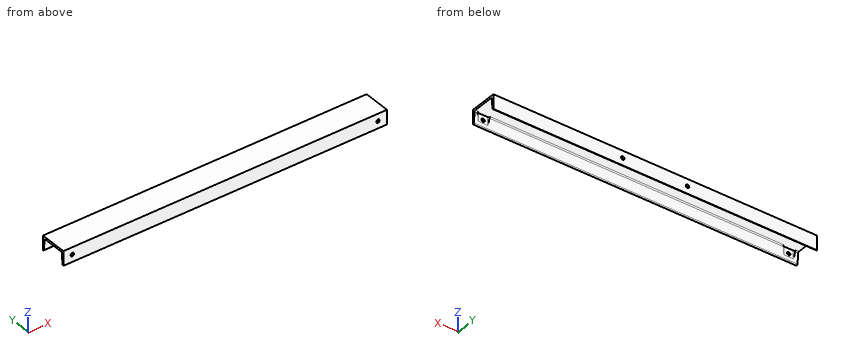
```python
from build123d import *

# Parameters (mm, degrees)
STRUCTURAL_MEMBER1_DEPTH = 900
SKETCH12_R               = 4.7625
CUT_EXTRUDE1_DEPTH       = 454.327971782
CUT_EXTRUDE2_DEPTH       = 40
SKETCH18_R               = 4.7625
CUT_EXTRUDE3_DEPTH       = 10


with BuildPart() as part:
    # Sketch17 → Structural Member1 (new body)
    with BuildSketch(Plane(origin=(-450, 0, 0), x_dir=(0, 0, 1), z_dir=(1, 0, 0))):
        with BuildLine():
            Line((0, 37.5), (0, -37.5))
            Line((0, -37.5), (-40, -37.5))
            Line((-40, -37.5), (-40, -37.246949676))
            ThreePointArc((-40, -37.246949676), (-39.212582687, -35.220998578), (-37.263681431, -34.258560126))
            Line((-37.263681431, -34.258560126), (-8.736318569, -31.741439874))
            ThreePointArc((-8.736318569, -31.741439874), (-6.787417313, -30.779001422), (-6, -28.753050324))
            Line((-6, -28.753050324), (-6, 28.753050324))
            ThreePointArc((-6, 28.753050324), (-6.787417313, 30.779001422), (-8.736318569, 31.741439874))
            Line((-8.736318569, 31.741439874), (-37.263681431, 34.258560126))
            ThreePointArc((-37.263681431, 34.258560126), (-39.212582687, 35.220998578), (-40, 37.246949676))
            Line((-40, 37.246949676), (-40, 37.5))
            Line((-40, 37.5), (0, 37.5))
        make_face()
    extrude(amount=STRUCTURAL_MEMBER1_DEPTH)

    # Sketch12 → Cut-Extrude1 (cut, through all)
    with BuildSketch(Plane(origin=(0, 0, 0), x_dir=(1, 0, 0), z_dir=(0, 1, 0))):
        with Locations(Location((-425, 20, 0), (0, 0, 270))):
            Circle(SKETCH12_R)
        with Locations(Location((425, 20, 0), (0, 0, 270))):
            Circle(SKETCH12_R)
    extrude(amount=-CUT_EXTRUDE1_DEPTH, mode=Mode.SUBTRACT)

    # Sketch15 → Cut-Extrude2 (cut)
    with BuildSketch(Plane(origin=(0, 0, -6), x_dir=(-1, 0, 0), z_dir=(0, 0, -1))):
        with BuildLine():
            Line((-412.5, -33.5), (-437.5, -33.5))
            ThreePointArc((-437.5, -33.5), (-442.5, -28.5), (-437.5, -23.5))
            Line((-437.5, -23.5), (-412.5, -23.5))
            ThreePointArc((-412.5, -23.5), (-407.5, -28.5), (-412.5, -33.5))
        make_face()
        with BuildLine():
            Line((412.5, -33.5), (437.5, -33.5))
            ThreePointArc((437.5, -33.5), (442.5, -28.5), (437.5, -23.5))
            Line((437.5, -23.5), (412.5, -23.5))
            ThreePointArc((412.5, -23.5), (407.5, -28.5), (412.5, -33.5))
        make_face()
    extrude(amount=CUT_EXTRUDE2_DEPTH, mode=Mode.SUBTRACT)

    # Sketch18 → Cut-Extrude3 (cut)
    with BuildSketch(Plane(origin=(0, 37.5, 0), x_dir=(1, 0, 0), z_dir=(0, 1, 0))):
        with Locations(Location((90, 20, 0), (0, 0, 270))):
            Circle(SKETCH18_R)
        with Locations(Location((-90, 20, 0), (0, 0, 270))):
            Circle(SKETCH18_R)
    extrude(amount=-CUT_EXTRUDE3_DEPTH, mode=Mode.SUBTRACT)


solid = part.part
```
Read the model definition and answer for the solid it produces. Units are mm, in the model's axes. Give positions to 0.01 mm unless a question says otherwise; leave off trailing zeros. Write each loop counter-clockwise with the first axis right and the second up, starting at its lowest first coordinate (ties: lowest second). Pieces come first, ordered by that corner, then holes. Notation, with made-up numbers: (-29.5, -12.5) - (16.5, -12.5) arc R28 ccw to (16.5, 18.5) - close; hole circle Ø3 at (7.5, 23). An arc over 180 degrees is marked (long way). Write item = value, one per line. Start each with the question number.
Item 1: Each of these flat-tipped pins is pushed along its axis until it touches: P1, Ø1, axis at x = 193.5, y = -9, coming from the -Z side; P2, Ø10, axis at y = -26.5, z = -24.5, coming from the +X side. Where does it stop, or does it pass through?
Item 2: Find section A-A (x = -236.5). Give the vertices of the cut face in (y, z).
Item 3: Find section B-B (y = 4). Give the vertices of the cut face in (x, z).
Item 4: Find the intervals of material crossed by probe 1 along X at (y, z) = (-34.5, -20); probe 2 along X at (y, z) = (34.1, -20); probe 3 along Y at (x, z) = (-94, -9), in increasing order. Write a range as [from, to].
Response:
q1.P1 = -6
q1.P2 = through
q2.outline = (-37.5, -40) - (-37.25, -40) arc R3 ccw to (-34.26, -37.26) - (-31.74, -8.74) arc R3 cw to (-28.75, -6) - (28.75, -6) arc R3 cw to (31.74, -8.74) - (34.26, -37.26) arc R3 ccw to (37.25, -40) - (37.5, -40) - (37.5, 0) - (-37.5, 0) - close
q3.outline = (-450, -6) - (450, -6) - (450, 0) - (-450, 0) - close
q4.probe_1 = [-450, -429.76], [-420.24, 420.24], [429.76, 450]
q4.probe_2 = [-450, -94.76], [-85.24, 85.24], [94.76, 450]
q4.probe_3 = [-37.5, -31.76], [31.76, 37.5]
